Design review of the part built by this model. Coordinates are the model's own, in mm. A direction names the side the tool comes from. Round coordinates to 2 decimals unless told otherwise and drop trailing zeros. Write each loop counter-clockwise with the first axis right and the second up, starting at its lowest first coordinate (ties: lowest second). Pieces come first, ordered by that corner, then holes. Notation, with made-up numbers: (-18, 6.5) - (40, 6.5) arc R25 cw to (40, 32.5) - close; hole circle Ø6 at (44.5, 33). An arc over 180 degrees is marked (long way). Use one line per item in the form item = value.
Autodesk Inventor part; units mm, degrees
ref_plane "YZ Plane" through (0, 0, 0) normal (1, 0, 0) x (0, 1, 0)
ref_plane "XZ Plane" through (0, 0, 0) normal (0, 1, 0) x (-1, 0, 0)
ref_plane "XY Plane" through (0, 0, 0) normal (0, 0, 1) x (1, 0, 0)
sketch "Skizze1" plane through (0, 0, 0) normal (1, 0, 0) x (0, 1, 0)
  line L0 (0, 0) -> (144, 0)
  line L1 (144, 0) -> (144, -68)
  line L2 (144, -68) -> (0, -68)
  line L3 (0, -68) -> (0, 0)
  dimension "d0" = 144
  dimension "d1" = 68
extrude "Extrusion1" add sketch "Skizze1" along normal blind 16
sketch "Skizze2" plane through (0, 0, 0) normal (0, 0, 1) x (1, 0, 0)
  line L0 (0, 0) -> (0, 144) construction
  line L1 (0, 72) -> (16, 72) construction
  line L2 (16, 144) -> (16, 0) construction
  line L3 (0, 144) -> (16, 144) construction
  line L4 (8, 144) -> (8, 0) construction
  line L5 (0, 144) -> (16, 144) construction
  line L6 (0, 0) -> (16, 0) construction
  line L7 (0, 144) -> (16, 144) construction
  line L8 (16, 144) -> (16, 0) construction
  line L9 (16, 0) -> (0, 0) construction
  line L10 (0, 0) -> (0, 144) construction
  line L11 (0, 112) -> (16, 112) construction
  line L12 (0, 32) -> (16, 32) construction
  point P0 (8, 112)
  point P1 (8, 72)
  point P2 (8, 32)
  dimension "d4" = 40
  dimension "d5" = 40
hole "Bohrung1" at (8, 112, 0) at (8, 72, 0) at (8, 32, 0) direction (0, 0, -1) diameter 3 depth 30 tip angle 118
sketch "Skizze3" plane through (0, 144, 0) normal (0, 1, 0) x (1, 0, 0)
  line L0 (0, 0) -> (16, 0)
  line L1 (16, 0) -> (16, 68)
  line L2 (16, 68) -> (0, 68)
  line L3 (0, 68) -> (0, 0)
  line L4 (8, 0) -> (8, 68) construction
  line L5 (0, 68) -> (16, 68) construction
  line L6 (16, 0) -> (16, 68) construction
  line L7 (16, 34) -> (0, 34) construction
  line L8 (0, 68) -> (0, 0) construction
  line L9 (0, 14) -> (16, 14) construction
  line L10 (0, 54) -> (16, 54) construction
  point P0 (8, 14)
  point P1 (8, 54)
  dimension "d13" = 14
  dimension "d22" = 14
hole "Bohrung2" at (8, 144, -14) at (8, 144, -54) direction (0, -1, 0) diameter 3 depth 25 tip angle 118
sketch "Skizze4" plane through (0, 0, -68) normal (0, 0, -1) x (-1, 0, 0)
  line L0 (0, 0) -> (-16, 0) construction
  line L1 (-16, 0) -> (-16, 144) construction
  line L2 (-16, 144) -> (0, 144) construction
  line L3 (0, 144) -> (0, 0) construction
  line L4 (-8, 0) -> (-8, 144) construction
  line L5 (-16, 144) -> (-16, 0) construction
  line L6 (-16, 72) -> (0, 72) construction
  circle A0 centre (-8, 72) radius 1.5 construction
  point P0 (-8, 112)
  point P1 (-8, 32)
  dimension "d23" = 40
  dimension "d24" = 40
hole "Bohrung3" at (8, 72, -68) at (8, 112, -68) at (8, 32, -68) direction (0, 0, 1) diameter 3 depth 30 tip angle 118
sketch "Skizze6" plane through (0, 0, 0) normal (-1, 0, 0) x (0, 0, 1)
  line L0 (0, 0) -> (-68, 0) construction
  line L1 (-68, 0) -> (-68, 144) construction
  line L2 (-68, 144) -> (0, 144) construction
  line L3 (0, 144) -> (0, 0) construction
  line L4 (0, 144) -> (0, 0) construction
  line L5 (0, 72) -> (-68, 72) construction
  line L6 (-68, 70.5) -> (-68, 73.5) construction
  line L7 (0, 0) -> (-68, 0) construction
  line L8 (-34, 0) -> (-34, 144) construction
  line L9 (0, 144) -> (-68, 144) construction
  line L10 (-25, 82) -> (-25, 62) construction
  point P0 (-25, 72)
  dimension "d41" = 25
  dimension "d42" = 10
hole "Bohrung5" at (0, 82, -25) at (0, 62, -25) direction (1, 0, 0) diameter 3 end through all countersink diameter 8 countersink angle 90
equation "\"d48\" = Stärke"
equation "\"Biegeradius\" = Stärke"
equation "\"BreiteBiegungsfreistellung\" = Stärke"
equation "\"TiefeBiegungsfreistellung\" = 0.5 * Stärke"
equation "\"GrößeEckenfreistellung\" = 4 * Stärke"
equation "\"MinimalRest\" = 2 * Stärke"
equation "\"Übergangsradius\" = Biegeradius"
equation "\"JacobiRadiusGröße\" = Biegeradius"
equation "\"Abstandsgröße\" = Stärke"
properties part number "licht_200_side_left"
Q1. Draft analysis for pull direction X (two halves, no side actions). For faces 4 (the conical face through (2.34, 63.4, -24.11)), 5 (the flat face through (8, 0, -34)), 6 (the conical face through (8.011, 31.74, -37.255)), state which applies: released by +X, released by -X, zero draft, split by the parting line, or undercut.
Calculated:
face_4 = released by -X
face_5 = zero draft
face_6 = undercut
Q2. We need section A-A on z = -25. Write out the cut boundary in (x, y).
Calculated:
outline = (0, 0) - (16, 0) - (16, 60.5) - (2.5, 60.5) - (0, 58) - close; (0, 66) - (2.5, 63.5) - (16, 63.5) - (16, 80.5) - (2.5, 80.5) - (0, 78) - close; (0, 86) - (2.5, 83.5) - (16, 83.5) - (16, 144) - (0, 144) - close; hole circle Ø3 at (8, 32); hole circle Ø3 at (8, 72); hole circle Ø3 at (8, 112)
Q3. We need section B-B on y = 62. Write out the cut boundary in (x, z), then the cut area to 3 significant figures.
Calculated:
outline = (0, -68) - (16, -68) - (16, -26.5) - (2.5, -26.5) - (0, -29) - close; (0, -21) - (2.5, -23.5) - (16, -23.5) - (16, 0) - (0, 0) - close
area = 1,030 mm2
Q4. To check wall thickness, follow line 1 along Y through (x, z) = (8, -10); line 2 along Z through (x, y) = (8, 126.5); line 3 along Y through (x, z) = (13.25, -25). State the ranges of each line that lie inside material, in increasing order. Write a range as from..to.
Calculated:
line_1 = 0..30.5, 33.5..70.5, 73.5..110.5, 113.5..144
line_2 = -68..-55.5, -52.5..-15.5, -12.5..0
line_3 = 0..60.5, 63.5..80.5, 83.5..144
Q5. For P1, Ø1.8, axis at x = 8, y = 112, coming from the -Z side; P2, Ø2.5, axis at x = 8, y = 72, coming from the -Z side, all flat-tipped, find the tip position at first contact; note any pin that passes through.
Calculated:
P1 = -37.64
P2 = -37.85
Q6. Machinability: for faces 1 (the cylindrical face through (7.93, 110.5, -52.79)), 2 (the flat face through (0, 71, -34)), 3 (the cylindrical face through (8.9, 131.3, -15.2)), which of the approach directions +Z, -Z, +X, -X, +Y, -Y give a long, thin tool a straight path to every point of the face, cutting with its end or side? Answer none if there is none.
Calculated:
face_1 = -Z
face_2 = +Z, -Z, -X, +Y, -Y
face_3 = +Y
